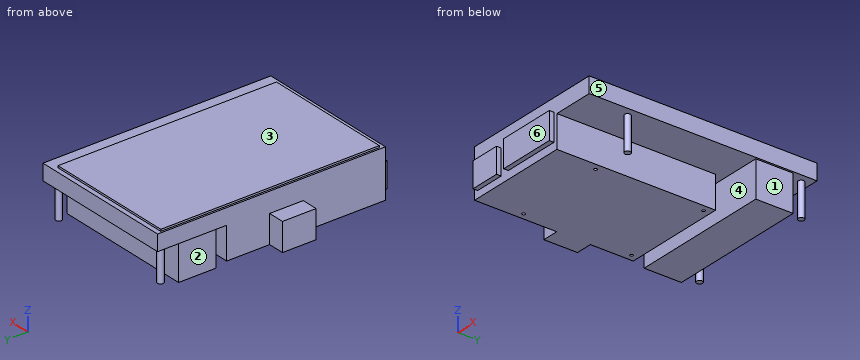
```python
from build123d import *

# Parameters (mm, degrees)
F0_W      = 78
F0_H      = 122
F1_DEPTH  = 8.5
F2_W      = 70
F2_H      = 117
F3_DEPTH  = 1
F4_W      = 56
F4_H      = 85
F5_DEPTH  = 17.25
F6_W      = 18
F6_H      = 15
F7_DEPTH  = 8.75
F8_W      = 16
F8_H      = 13.5
F8_W_2    = 31
F8_H_2    = 14.5
F9_DEPTH  = 2.5
F10_R     = 0.8
F11_DEPTH = 5
F12_R     = 1.6
F13_DEPTH = 18
F14_W     = 76
F14_H     = 20
F15_DEPTH = 19.4


with BuildPart() as f1:
    # F0 (on Top) → F1 (new body)
    with BuildSketch(Plane.XY):
        Rectangle(F0_W, F0_H)
    extrude(amount=F1_DEPTH)

    # F2 (on face) → F3 (join)
    with BuildSketch(Plane.XY.offset(8.5)):
        with Locations((-3, 0)):
            Rectangle(F2_W, F2_H)
    extrude(amount=F3_DEPTH)

    # F4 (on face) → F5 (join)
    with BuildSketch(Plane(origin=(0, 0, 0), x_dir=(1, 0, 0), z_dir=(0, 0, -1))):
        with Locations((-11, 18.5)):
            Rectangle(F4_W, F4_H)
    extrude(amount=F5_DEPTH)

    # F6 (on face) → F7 (join)
    with BuildSketch(Plane(origin=(-39, 0, 0), x_dir=(0, -1, 0), z_dir=(-1, 0, 0))):
        with Locations((8, -9.75)):
            Rectangle(F6_W, F6_H)
    extrude(amount=F7_DEPTH)

    # F8 (on face) → F9 (join)
    with BuildSketch(Plane.XZ.offset(61)):
        with Locations((-28.9, -6.75)):
            Rectangle(F8_W, F8_H)
        with Locations((-0.5, -5.75)):
            Rectangle(F8_W_2, F8_H_2)
    extrude(amount=F9_DEPTH)

    # F10 (on face) → F11 (cut)
    with BuildSketch(Plane(origin=(0, 0, -17.25), x_dir=(1, 0, 0), z_dir=(0, 0, -1))):
        with Locations((13.5, 37.5)):
            Circle(F10_R)
        with Locations((-35.5, 37.5)):
            Circle(F10_R)
        with Locations((-35.5, -20.35)):
            Circle(F10_R)
        with Locations((13.5, -20.35)):
            Circle(F10_R)
    extrude(amount=-F11_DEPTH, mode=Mode.SUBTRACT)

    # F12 (on face) → F13 (join)
    with BuildSketch(Plane(origin=(0, 0, 0), x_dir=(1, 0, 0), z_dir=(0, 0, -1))):
        with Locations((-35.1, -56.4)):
            Circle(F12_R)
        with Locations((34.1, -56.4)):
            Circle(F12_R)
        with Locations((34.1, 36.6)):
            Circle(F12_R)
    extrude(amount=F13_DEPTH)

    # F14 (on face) → F15 (join)
    with BuildSketch(Plane(origin=(0, 0, 0), x_dir=(1, 0, 0), z_dir=(0, 0, -1))):
        with Locations((0, -39)):
            Rectangle(F14_W, F14_H)
    extrude(amount=F15_DEPTH)


solid = f1.part
```
The listing builds one solid part. Answer for the finished solid, in the listing's coordinates (mm). Face numbers are marked on the shaded views. A direction names the side the tool comes from. Round coordinates to 2 decimals unless told otherwise and drop trailing zeros. Loops run counter-clockwise (first coordinate to the right, second up) from the corner with the lowest first, then second, coordinate; pieces in that order, holes last. Notation, with made-up numbers: (14.25, -22.75) - (69.25, -22.75) arc R14 ccw to (69.25, -12.75) - close; hole circle Ø2 at (19, 27.5). An arc over 180 degrees is marked (long way). Use one line per item in the form item = value. Start each with the question number.
1. The part is cut by section B-B on x = -6. Determine the outline of the cut face in (y, z), then the cut area to 3 significant figures.
2. Consider line 1 (X direction, y = 20.35, z = -16.15); line 2 (Y direction, x = 13.5, z = -14.45); line 3 (Y direction, x = -28.5, z = -8.5). Determine where each line is inside the solid, lowest interval first. Write a range as [from, to].
3. Given pin 1 Ø19.5 at (x, y) = (-6.5, -14.5) entering from -Z; pin 2 Ø9.5 at (x, z) = (-6, -7) entering from +Y; pin 3 Ø1.6 at (x, y) = (34.5, -36) entering from -Z, each flat-ended and moving along its own axis, determine where each tip first touches the part or whether it passes through.
4. The part is cut by section C-C on y = 6. Determine the outline of the cut face in (x, z), then the cut area to 3 significant figures.
5. A tool of negligible diameter and unlimited length cuts with its end or side. For the marked faces 1, 2 and 3, from which of +Z, -Z, +X, -X, +Y, -Y can it reach the whole face along a straight path? Write none if from no direction.
6. The part is cut by section D-D on y = 27. Determine the outline of the cut face in (x, z).
7. For a pull along Y with two mould halves and no side action, classify the marked faces 4, 5 and 6 as pulls with the +Y half, pulls with the -Y half, needs draft (parallel to the pull), parting line crosses it, or undercut.
8. The part is cut by section A-A on z = -4. Determine the outline of the cut face in (x, y).
Geometry check:
q1.outline = (-63.5, -13) - (-61, -13) - (-61, -17.25) - (24, -17.25) - (24, 0) - (29, 0) - (29, -19.4) - (49, -19.4) - (49, 0) - (61, 0) - (61, 8.5) - (58.5, 8.5) - (58.5, 9.5) - (-58.5, 9.5) - (-58.5, 8.5) - (-61, 8.5) - (-61, 1.5) - (-63.5, 1.5) - close
q1.area = 3,040 mm^2
q2.line_1 = [-39, -36.3], [-34.7, 12.7], [14.3, 17]
q2.line_2 = [-61, -38.3], [-36.7, 19.55], [21.15, 24], [29, 49]
q2.line_3 = [-63.5, 24], [29, 49]
q3.pin_1 = -17.25
q3.pin_2 = 49
q3.pin_3 = -18
q4.outline = (-39, -17.25) - (17, -17.25) - (17, 0) - (39, 0) - (39, 8.5) - (32, 8.5) - (32, 9.5) - (-38, 9.5) - (-38, 8.5) - (-39, 8.5) - close
q4.area = 1,700 mm^2
q5.face_1 = -Z, +X, +Y, -Y
q5.face_2 = -Z, -X, +Y
q5.face_3 = +Z, +X, -X, +Y, -Y
q6.outline = (-39, 0) - (39, 0) - (39, 8.5) - (32, 8.5) - (32, 9.5) - (-38, 9.5) - (-38, 8.5) - (-39, 8.5) - close
q7.face_4 = undercut
q7.face_5 = needs draft
q7.face_6 = pulls with the -Y half
q8.outline = (-47.75, -17) - (-39, -17) - (-39, -61) - (-36.9, -61) - (-36.9, -63.5) - (-20.9, -63.5) - (-20.9, -61) - (-16, -61) - (-16, -63.5) - (15, -63.5) - (15, -61) - (17, -61) - (17, 24) - (-39, 24) - (-39, 1) - (-47.75, 1) - close; (-38, 29) - (38, 29) - (38, 49) - (-38, 49) - close; circle Ø3.2 at (-35.1, 56.4); circle Ø3.2 at (34.1, -36.6); circle Ø3.2 at (34.1, 56.4)
